Verification items for this drawing (mm, ordinates from the low corner). Coordinates: 2 decimals unless noted, no trailing zeros. Write each loop counter-clockwise with the first axis right and the second up, starting at its lowest first coordinate (ties: lowest second). Pieces come first, ordered by that corner, then holes. Notation, with made-up numbers: M 70.5,20.25 L 109.5,20.25 A22 cw 109.5,58.25 Z; hole C 22,62.5 d4. An arc over 180 degrees is marked long. Put each result on its own line as item: value. Start each with the question number.
1) Cross-section at A-A on x = 65.5. Record the cut outline in (y, z), plus the area to 3 significant figures.
2) Gauge pin test, flat ends, axial feed: pin 1 (1.5 mm diameter, centred on y = 3.5, z = 2, fed in from +X); pin 2 (1.5 mm diameter, centred on x = 5.5, y = 3, fed in from -Z); pin 3 (1.5 mm diameter, centred on x = 95.5, y = 2, fed in from +Z). Record the tip position at first contact, or that the pin passes through.
3) Scan lines: line 1 along Z through (x, y) = (65.5, 1.7); line 2 along X through (y, z) = (1.6, 33.5); line 3 along Z through (x, y) = (25, 3.1). Record each from-to range of solid material in increasing order.
4) Cross-section at B-B on z = 49. Record the cut outline in (x, y), plus the area to 3 significant figures.
5) Cross-section at C-C on x = 25. Record the cut outline in (y, z).
6) Cross-section at D-D on z = 33.5. Record the cut outline in (x, y), plus the area to 3 significant figures.
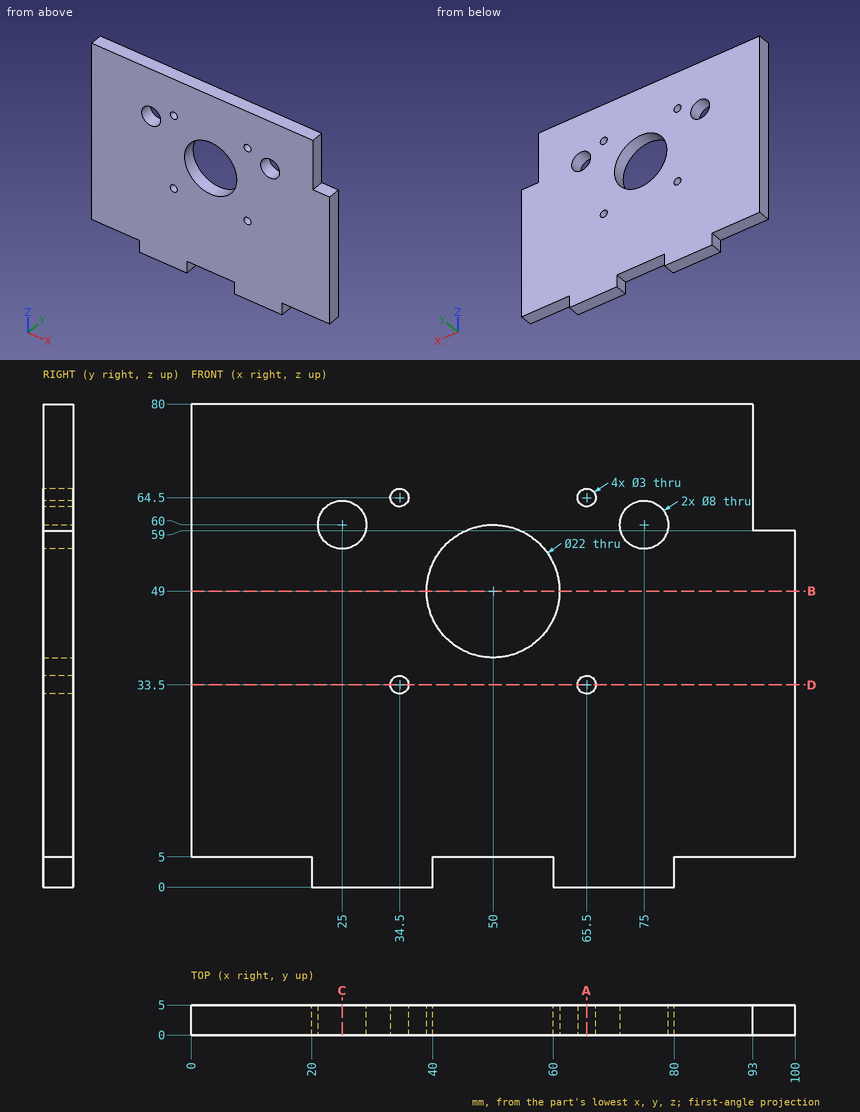
Answer key:
1. outline: M 0,0 L 5,0 L 5,32 L 0,32 Z; M 0,35 L 5,35 L 5,63 L 0,63 Z; M 0,66 L 5,66 L 5,80 L 0,80 Z
1. area: 370 mm²
2. pin 1: stops at x = 80
2. pin 2: stops at z = 5
2. pin 3: stops at z = 59
3. line 1: z = 0 to 32, 35 to 63, 66 to 80
3. line 2: x = 0 to 33, 36 to 64, 67 to 100
3. line 3: z = 0 to 56, 64 to 80
4. outline: M 0,0 L 39,0 L 39,5 L 0,5 Z; M 61,0 L 100,0 L 100,5 L 61,5 Z
4. area: 390 mm²
5. outline: M 0,0 L 5,0 L 5,56 L 0,56 Z; M 0,64 L 5,64 L 5,80 L 0,80 Z
6. outline: M 0,0 L 33,0 L 33,5 L 0,5 Z; M 36,0 L 64,0 L 64,5 L 36,5 Z; M 67,0 L 100,0 L 100,5 L 67,5 Z
6. area: 470 mm²
